Geometry check sheet. Reference: the model listing, model coordinates, mm. Coordinates: 2 decimals unless noted, no trailing zeros. Loops run counter-clockwise (first coordinate to the right, second up) from the corner with the lowest first, then second, coordinate; pieces in that order, holes last. Notation, with made-up numbers: M 22.25,13 L 29.25,13 A22 cw 29.25,37 Z; hole C 43.5,23.5 d5. An arc over 180 degrees is marked long. Use CSV: the item, a comma, the result in double quotes.
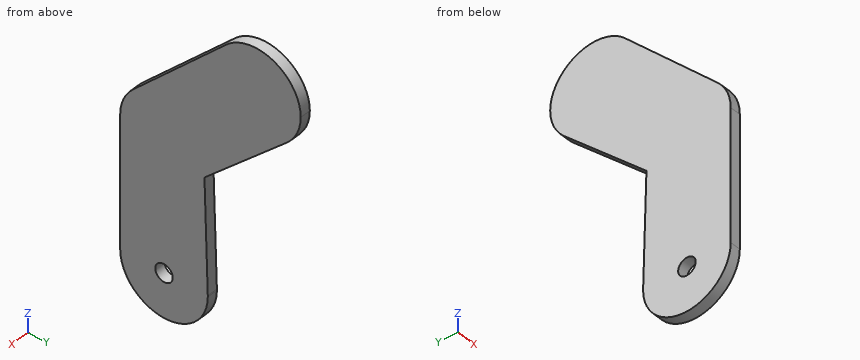
```python
from build123d import *

# Parameters (mm, degrees)
F1_DEPTH = 6
F2_R     = 5
F3_DEPTH = 6


with BuildPart() as f1:
    # F0 (on Right) → F1 (new body)
    with BuildSketch(Plane.YZ):
        with BuildLine():
            ThreePointArc((-25, 0), (0, -25), (25, 0))
            ThreePointArc((25, 0), (24.997328528, 0.3654674576), (24.989314683, 0.7308568083))
            ThreePointArc((24.989314683, 0.7308568083), (17.4173559961, 17.9342050313), (0, 25))
            ThreePointArc((0, 25), (-17.6776695297, 17.6776695297), (-25, 0))
        make_face()
        with BuildLine():
            ThreePointArc((0, 25), (17.4173559961, 17.9342050313), (24.989314683, 0.7308568083))
            Line((24.989314683, 0.7308568083), (23.0969883128, 65.4329141909))
            ThreePointArc((23.0969883128, 65.4329141909), (13.8892558255, 54.2132596924), (0, 50))
            Line((0, 50), (0, 25))
        make_face()
        with BuildLine():
            Line((-25, 75), (-25, 0))
            ThreePointArc((-25, 0), (-17.6776695297, 17.6776695297), (0, 25))
            Line((0, 25), (0, 50))
            ThreePointArc((0, 50), (-17.6776695297, 57.3223304703), (-25, 75))
        make_face()
        with BuildLine():
            Line((0, 75), (23.0969883128, 65.4329141909))
            ThreePointArc((23.0969883128, 65.4329141909), (24.5196320101, 70.1227419496), (25, 75))
            ThreePointArc((25, 75), (23.0969883128, 84.5670858091), (17.6776695297, 92.6776695297))
            Line((17.6776695297, 92.6776695297), (0, 75))
        make_face()
        with BuildLine():
            ThreePointArc((0, 50), (13.8892558255, 54.2132596924), (23.0969883128, 65.4329141909))
            Line((23.0969883128, 65.4329141909), (0, 75))
            Line((0, 75), (0, 50))
        make_face()
        with BuildLine():
            ThreePointArc((25, 75), (24.5196320101, 70.1227419496), (23.0969883128, 65.4329141909))
            Line((23.0969883128, 65.4329141909), (70.1863286533, 109.8461009142))
            ThreePointArc((70.1863286533, 109.8461009142), (52.6675411314, 103.035680061), (35.3553390593, 110.3553390593))
            Line((35.3553390593, 110.3553390593), (17.6776695297, 92.6776695297))
            ThreePointArc((17.6776695297, 92.6776695297), (23.0969883128, 84.5670858091), (25, 75))
        make_face()
        with BuildLine():
            ThreePointArc((-17.6737877377, 92.6815504694), (-23.0959378836, 84.569621376), (-25, 75))
            ThreePointArc((-25, 75), (-17.6776695297, 57.3223304703), (0, 50))
            Line((0, 50), (0, 75))
            Line((0, 75), (17.6776695297, 92.6776695297))
            ThreePointArc((17.6776695297, 92.6776695297), (0.0027445402, 99.9999998493), (-17.6737877377, 92.6815504694))
        make_face()
        with BuildLine():
            ThreePointArc((35.3553390593, 110.3553390593), (52.6675411314, 103.035680061), (70.1863286533, 109.8461009142))
            ThreePointArc((70.1863286533, 109.8461009142), (75.9876704424, 118.1292972041), (78.033008589, 128.033008589))
            ThreePointArc((78.033008589, 128.033008589), (62.1819121392, 151.298811043), (34.7292034826, 145.0615352026))
            ThreePointArc((34.7292034826, 145.0615352026), (28.0370760813, 127.5820561841), (35.3553390593, 110.3553390593))
        make_face()
        with BuildLine():
            Line((34.7292034826, 145.0615352026), (-17.6737877377, 92.6815504694))
            ThreePointArc((-17.6737877377, 92.6815504694), (0.0027445402, 99.9999998493), (17.6776695297, 92.6776695297))
            Line((17.6776695297, 92.6776695297), (35.3553390593, 110.3553390593))
            ThreePointArc((35.3553390593, 110.3553390593), (28.0370760813, 127.5820561841), (34.7292034826, 145.0615352026))
        make_face()
    extrude(amount=F1_DEPTH)

    # F2 (on face) → F3 (cut)
    with BuildSketch(Plane.YZ.offset(6)):
        Circle(F2_R)
    extrude(amount=-F3_DEPTH, mode=Mode.SUBTRACT)


solid = f1.part
```
1. Section check B-B, the plane y = 0. Record the cut outline in (x, z), plus the area to 3 significant figures.
The answers:
outline,"M 0,-25 L 6,-25 L 6,-5 L 0,-5 Z; M 0,5 L 6,5 L 6,110.35 L 0,110.35 Z"
area,"752 mm^2"
2. Section check C-C, the plane z = -2.5. Record the cut outline in (x, y).
The answers:
outline,"M 0,-24.87 L 6,-24.87 L 6,-4.33 L 0,-4.33 Z; M 0,4.33 L 6,4.33 L 6,24.87 L 0,24.87 Z"
3. Section check A-A, the plane x = 3.75. Record the cut outline in (y, z), plus the area to 3 significant figures.
The answers:
outline,"M -25,0 A25 ccw long 24.99,0.73 L 23.1,65.43 L 70.19,109.85 A25 ccw long 34.73,145.06 L -17.67,92.68 A25 ccw -25,75 Z; hole C 0,0 d10"
area,"9,250 mm^2"
4. Gauge pin test, flat ends, axial feed: P1, Ø3, axis at y = 20, z = 15, coming from the -X side; P2, Ø3, axis at x = 1.5, y = -6.5, coming from the -Z side. Record the tip position at first contact, or that the pin passes through.
The answers:
P1,"x = 0"
P2,"z = -24.49"
5. Thickness scan on line 1 (Z direction, x = 2.1, y = 0); line 2 (Y direction, x = 4.55, z = 2); line 3 (Z direction, x = 1.2, y = 12). Record the ranges inside material, lowest first. Write a range as [from, to].
The answers:
line 1,"[-25, -5], [5, 110.35]"
line 2,"[-25, -4.58], [4.58, 24.95]"
line 3,"[-21.93, 122.34]"
6. Section check D-D, the plane z = 106.5. Record the cut outline in (x, y), plus the area to 3 significant figures.
The answers:
outline,"M 0,-3.85 L 6,-3.85 L 6,66.64 L 0,66.64 Z"
area,"423 mm^2"
